Autodesk Inventor part; units mm, degrees
ref_plane "YZ Plane" through (0, 0, 0) normal (1, 0, 0) x (0, 1, 0)
ref_plane "XZ Plane" through (0, 0, 0) normal (0, 1, 0) x (-1, 0, 0)
ref_plane "XY Plane" through (0, 0, 0) normal (0, 0, 1) x (1, 0, 0)
sketch "Sketch1" plane through (0, 0, 0) normal (0, 1, 0) x (-1, 0, 0)
  line L0 (0, 0) -> (-152.4, 0)
  line L1 (-152.4, 0) -> (-152.4, -127)
  line L2 (-152.4, -127) -> (0, -127)
  line L3 (0, -127) -> (0, 0)
  line L4 (0, 0) -> (-152.4, 0)
  line L5 (-152.4, 0) -> (-152.4, 3.175)
  line L6 (-152.4, 3.175) -> (0, 3.175)
  line L7 (0, 3.175) -> (0, 0)
  line L8 (0, -127) -> (-152.4, -127)
  line L9 (-152.4, -127) -> (-152.4, -130.175)
  line L10 (-152.4, -130.175) -> (0, -130.175)
  line L11 (0, -130.175) -> (0, -127)
  dimension "d0" = 152.4
  dimension "d1" = 127
  dimension "d2" = 152.4
  dimension "d3" = 3.175
  dimension "d4" = 152.4
  dimension "d5" = 3.175
extrude "Extrusion1" add sketch "Sketch1" along normal blind 50.8 contours L0 L5 L6 L7 | L11 L10 L9 L2
sketch "Sketch2" plane through (0, 50.8, 0) normal (0, 1, 0) x (1, 0, 0)
  line L0 (0, -3.175) -> (152.4, -3.175)
  line L1 (0, -3.175) -> (-3.175, -3.175)
  line L2 (-3.175, -3.175) -> (-3.175, 130.175)
  line L3 (-3.175, 130.175) -> (0, 130.175)
  line L4 (0, 130.175) -> (0, -3.175)
  point P0 (0, 0)
  dimension "d8" = 3.175
  dimension "d9" = 133.35
extrude "Extrusion2" add sketch "Sketch2" against normal blind 45.72
sketch "Sketch3" plane through (0, 0, 3.175) normal (0, 0, 1) x (1, 0, 0)
  line L0 (-3.175, 5.08) -> (0, 5.08)
  line L1 (-3.175, 5.08) -> (0, 5.08)
  line L2 (0, 5.08) -> (0, 0)
  line L3 (0, 0) -> (-3.175, 0)
  line L4 (-3.175, 0) -> (-3.175, 5.08)
extrude "Extrusion3" add sketch "Sketch3" against normal blind 3.175
sketch "Sketch4" plane through (152.4, 0, -130.175) normal (0, 0, -1) x (-1, 0, 0)
  line L0 (152.4, 0) -> (155.575, 0)
  line L1 (155.575, 0) -> (155.575, 5.08)
  line L2 (155.575, 5.08) -> (152.4, 5.08)
  line L3 (152.4, 5.08) -> (152.4, 0)
extrude "Extrusion4" add sketch "Sketch4" against normal blind 3.175
sketch "Sketch5" plane through (0, 50.8, 0) normal (0, 1, 0) x (1, 0, 0)
  line L0 (152.4, -3.175) -> (152.4, 0)
  line L1 (0, 127) -> (152.4, 127)
  line L2 (152.4, 0) -> (149.225, 0)
  line L3 (149.225, 0) -> (149.225, 127)
  line L4 (149.225, 127) -> (152.4, 127)
  line L5 (152.4, 127) -> (152.4, 0)
  point P0 (0, 0)
  dimension "d16" = 3.175
extrude "Extrusion5" add sketch "Sketch5" against normal blind 45.72
sketch "Sketch7" plane through (0, 0, 0) normal (0, -1, 0) x (1, 0, 0)
  line L0 (-3.175, 3.175) -> (-3.175, 0)
  line L1 (152.4, -127) -> (152.4, 0)
  line L2 (-3.175, 3.175) -> (152.4, 3.175)
  line L3 (152.4, 3.175) -> (152.4, -9.525)
  line L4 (152.4, -9.525) -> (-3.175, -9.525)
  line L5 (-3.175, -9.525) -> (-3.175, 3.175)
  line L6 (-3.175, -130.175) -> (-3.175, 3.175)
  line L7 (-3.175, -130.175) -> (152.4, -130.175)
  line L8 (152.4, -130.175) -> (152.4, -117.475)
  line L9 (152.4, -117.475) -> (-3.175, -117.475)
  line L10 (-3.175, -117.475) -> (-3.175, -130.175)
  point P0 (0, 0)
  point P1 (-3.175, -117.475)
  dimension "d19" = 12.7
  dimension "d20" = 155.575
  dimension "d21" = 12.7
extrude "Extrusion6" add sketch "Sketch7" along normal blind 3.175 contours L2 L3 L1 L4 L5 L0 | L9 L1 L8 L7 L6
sketch "Sketch8" plane through (0, 50.8, 0) normal (0, 1, 0) x (1, 0, 0)
  line L0 (0, 0) -> (49.53, 0) construction
  line L1 (49.53, 0) -> (49.53, 127) construction
  line L2 (49.53, 127) -> (0, 127) construction
  line L3 (0, 127) -> (0, 0) construction
  line L4 (149.225, 0) -> (152.4, 0) construction
  line L5 (149.225, 0) -> (99.695, 0) construction
  line L6 (99.695, 0) -> (99.695, 127) construction
  line L7 (99.695, 127) -> (149.225, 127) construction
  line L8 (149.225, 127) -> (149.225, 0) construction
  line L9 (99.695, 0) -> (96.52, 0)
  line L10 (96.52, 0) -> (96.52, 127)
  line L11 (96.52, 127) -> (99.695, 127)
  line L12 (99.695, 127) -> (99.695, 0)
  line L13 (49.53, 0) -> (52.705, 0)
  line L14 (52.705, 0) -> (52.705, 127)
  line L15 (52.705, 127) -> (49.53, 127)
  line L16 (49.53, 127) -> (49.53, 0)
  dimension "d24" = 49.53
  dimension "d25" = 127
  dimension "d26" = 49.53
  dimension "d27" = 127
  dimension "d28" = 3.175
  dimension "d29" = 127
  dimension "d30" = 3.175
  dimension "d31" = 127
extrude "Extrusion7" add sketch "Sketch8" against normal blind 45.72
sketch "Sketch9" plane through (152.4, 50.8, 3.175) normal (1, 0, 0) x (0, 0, -1)
  line L0 (0, 0) -> (133.35, 0)
  line L1 (133.35, 0) -> (133.35, 50.8)
  line L2 (133.35, 50.8) -> (0, 50.8)
  line L3 (0, 50.8) -> (0, 0)
  line L4 (133.35, 50.8) -> (184.15, 50.8)
  line L5 (184.15, 50.8) -> (133.35, 0)
  line L6 (0, 50.8) -> (-50.8, 50.8)
  line L7 (0, 50.8) -> (50.8, 50.8) construction
  line L8 (-50.8, 50.8) -> (0, 0)
  point P0 (3.175, -50.8)
  dimension "d34" = 133.35
  dimension "d35" = 50.8
  dimension "d36" = 50.8
  dimension "d37" = 50.8
  dimension "d38" = 180
extrude "Extrusion8" add sketch "Sketch9" against normal blind 3.175
sketch "Sketch10" plane through (-3.175, 50.8, -130.175) normal (-1, 0, 0) x (0, 0, 1)
  line L0 (3.175, 0) -> (0, 0)
  line L1 (0, 0) -> (133.35, 0)
  line L2 (133.35, 0) -> (133.35, 50.8)
  line L3 (133.35, 50.8) -> (0, 50.8)
  line L4 (0, 50.8) -> (0, 0)
  line L5 (-50.8, 50.8) -> (184.15, 50.8)
  line L6 (0, 50.8) -> (-50.8, 50.8)
  line L7 (-50.8, 50.8) -> (0, 0)
  line L8 (133.35, 50.8) -> (184.15, 50.8)
  line L9 (133.35, 0) -> (184.15, 50.8)
  point P0 (130.175, -50.8)
  dimension "d41" = 133.35
  dimension "d42" = 50.8
extrude "Extrusion9" add sketch "Sketch10" against normal blind 3.175
sketch "Sketch11" plane through (-3.175, 50.8, 3.175) normal (0, -0.7071, 0.7071) x (1, 0, 0)
  line L0 (0, 71.842) -> (0, -94.2927)
  line L1 (155.575, 0) -> (155.575, -38.1661)
  line L2 (0, 71.842) -> (155.575, 71.842)
  line L3 (155.575, 71.842) -> (155.575, 0)
  line L4 (155.575, 0) -> (0, 0)
  line L5 (0, 0) -> (0, 71.842)
  point P0 (3.175, -38.1661)
  point P1 (0, 0)
extrude "Extrusion10" add sketch "Sketch11" along normal blind 3.175
sketch "Sketch12" plane through (152.4, 50.8, -130.175) normal (0, -0.7071, -0.7071) x (-1, 0, 0)
  line L0 (0, 0) -> (0, 71.842)
  line L1 (152.4, 0) -> (155.575, 0)
  line L2 (0, 71.842) -> (155.575, 71.842)
  line L3 (155.575, 71.842) -> (155.575, 0)
  line L4 (155.575, 0) -> (0, 0)
  line L5 (0, 0) -> (0, 71.842)
  point P0 (152.4, -127.9686)
extrude "Extrusion11" add sketch "Sketch12" along normal blind 3.175
sketch "Sketch13" plane through (-3.175, 101.6, 53.975) normal (0, 1, 0) x (1, 0, 0)
  line L0 (52.705, 180.975) -> (52.705, 53.975) construction
  line L1 (52.705, 53.975) -> (52.705, 0) construction
  line L2 (152.4, 0) -> (3.175, 0) construction
  line L3 (55.88, 53.975) -> (55.88, 180.975) construction
  line L4 (55.88, 180.975) -> (55.88, 234.95) construction
  line L5 (3.175, 234.95) -> (152.4, 234.95) construction
  line L6 (52.705, 0) -> (55.88, 0)
  line L7 (55.88, 0) -> (55.88, 234.95)
  line L8 (55.88, 234.95) -> (52.705, 234.95)
  line L9 (52.705, 234.95) -> (52.705, 0)
  point P0 (3.175, 53.975)
extrude "Extrusion12" add sketch "Sketch13" against normal blind 3.175
sketch "Sketch14" plane through (52.705, 101.6, 53.975) normal (1, 0, 0) x (0, 0, -1)
  line L0 (3.175, -3.175) -> (50.8, -50.8)
  line L1 (50.8, -50.8) -> (50.8, -3.175)
  line L2 (231.775, -3.175) -> (3.175, -3.175)
  point P0 (53.975, -101.6)
extrude "Extrusion13" add sketch "Sketch14" against normal blind 3.175
sketch "Sketch15" plane through (52.705, 101.6, 53.975) normal (1, 0, 0) x (0, 0, -1)
  line L0 (50.8, -50.8) -> (50.8, -3.175)
  line L1 (50.8, -3.175) -> (184.15, -3.175)
  line L2 (184.15, -3.175) -> (184.15, -50.8)
  line L3 (184.15, -50.8) -> (50.8, -50.8)
  line L4 (50.8, -50.8) -> (50.8, -3.175)
  line L5 (184.15, -50.8) -> (231.775, -3.175)
  line L6 (231.775, -3.175) -> (184.15, -3.175)
  line L7 (231.775, -3.175) -> (50.8, -3.175)
  point P0 (53.975, -101.6)
extrude "Extrusion14" add sketch "Sketch15" against normal blind 3.175
sketch "Sketch16" plane through (-3.175, 101.6, 53.975) normal (0, 1, 0) x (1, 0, 0)
  line L0 (152.4, 53.975) -> (102.87, 53.975) construction
  line L1 (102.87, 53.975) -> (102.87, 0) construction
  line L2 (152.4, 0) -> (55.88, 0) construction
  line L3 (55.88, 180.975) -> (99.695, 180.975) construction
  line L4 (99.695, 180.975) -> (99.695, 234.95) construction
  line L5 (55.88, 234.95) -> (152.4, 234.95) construction
  line L6 (102.87, 0) -> (99.695, 0)
  line L7 (99.695, 0) -> (99.695, 234.95)
  line L8 (99.695, 234.95) -> (102.87, 234.95)
  line L9 (102.87, 234.95) -> (102.87, 0)
  point P0 (3.175, 53.975)
extrude "Extrusion15" add sketch "Sketch16" against normal blind 3.175
sketch "Sketch17" plane through (99.695, 101.6, 53.975) normal (1, 0, 0) x (0, 0, -1)
  line L0 (231.775, -3.175) -> (3.175, -3.175)
  line L1 (3.175, -3.175) -> (50.8, -50.8)
  line L2 (50.8, -50.8) -> (50.8, -3.175)
  line L3 (50.8, -3.175) -> (3.175, -3.175)
  line L4 (50.8, -3.175) -> (184.15, -3.175)
  line L5 (184.15, -3.175) -> (184.15, -50.8)
  line L6 (184.15, -50.8) -> (50.8, -50.8)
  line L7 (50.8, -50.8) -> (50.8, -3.175)
  line L8 (184.15, -3.175) -> (231.775, -3.175)
  line L9 (184.15, -50.8) -> (231.775, -3.175)
  point P0 (53.975, -101.6)
extrude "Extrusion16" add sketch "Sketch17" against normal blind 3.175
properties part number "BeadCompartments_2"
Source: CAD feature listing. Evaluate the final solid. Frame: model axes, mm. A direction names the side the tool comes from. Coordinates: 2 decimals unless noted, no trailing zeros. Order: outer loops, then holes, each group sorted by start corner. A loop starts at its lowest first (then second) coordinate and runs counter-clockwise, first axis right, second up. Notation, with made-up numbers: (11, 22) - (56, 22) arc R29 ccw to (56, 43) - close; hole circle Ø2 at (42.5, 46). An arc over 180 degrees is marked (long way). One line per item, written item: value.
1) Cut plane C-C on y = 20. Output: boundary loops of the cut face in (x, z) (3 decimals), plus the area to 3 significant figures.
Computed values:
outline: (-3.175, -130.175) - (152.4, -130.175) - (152.4, 3.175) - (-3.175, 3.175) - close; hole (0, -127) - (49.53, -127) - (49.53, 0) - (0, 0) - close; hole (52.705, -127) - (96.52, -127) - (96.52, 0) - (52.705, 0) - close; hole (99.695, -127) - (149.225, -127) - (149.225, 0) - (99.695, 0) - close
area: 2,600 mm^2
2) Cut plane A-A on z = -58.5. Output: boundary loops of the cut face in (x, y) (3 decimals).
Computed values:
outline: (-3.175, 5.08) - (0, 5.08) - (0, 101.6) - (-3.175, 101.6) - close; (49.53, 5.08) - (52.705, 5.08) - (52.705, 101.6) - (49.53, 101.6) - close; (96.52, 5.08) - (99.695, 5.08) - (99.695, 101.6) - (96.52, 101.6) - close; (149.225, 5.08) - (152.4, 5.08) - (152.4, 101.6) - (149.225, 101.6) - close
3) Contact query for flat-ended pins moving along their axis: pin 1 (3.5 mm diameter, centred on x = 98.5, z = -73, fed in from -Y); pin 2 (1.6 mm diameter, centred on x = 38.5, y = -1, fed in from -Z) (3 decimals); pin 3 (8 mm diameter, centred on x = 45.5, z = -30, fed in from +Y); pin 4 (3.5 mm diameter, centred on x = 82, z = -128.5, fed in from +Y) (3 decimals). Output: stop coordinate, or through.
Computed values:
pin 1: stops at y = 5.08
pin 2: stops at z = -130.175
pin 3: passes through
pin 4: stops at y = 50.875
4) Ray query, line 1 (X direction, y = 72, z = 16) (3 decimals); line 2 (Z direction, x = 145, y = 43.5) (3 decimals); line 3 (Z direction, x = 88.5, y = 57.5) (3 decimals). Return the intervals inside material, ascending. Write a range as [from, to].
Computed values:
line 1: x = [-3.175, 0], [49.53, 52.705], [96.52, 99.695], [149.225, 152.4]
line 2: z = [-130.175, -127], [0, 3.175]
line 3: z = [-141.365, -136.875], [9.875, 14.365]
5) Reachability of faces 1 (the face through (73.523, 74.311, 31.176)), 2 (the face through (74.919, 76.556, -155.931)) from +Z, -Z, +X, -X, +Y, -Y: full face, straight path, thin tool, end or side. Return the list, or none.
Computed values:
face 1: +Z, +X, -X, -Y
face 2: +Y
6) Cut plane D-D on y = 91.5. Output: boundary loops of the cut face in (x, z) (3 decimals).
Computed values:
outline: (-3.175, -175.365) - (152.4, -175.365) - (152.4, 48.365) - (-3.175, 48.365) - close; hole (0, -170.875) - (49.53, -170.875) - (49.53, 43.875) - (0, 43.875) - close; hole (52.705, -170.875) - (96.52, -170.875) - (96.52, 43.875) - (52.705, 43.875) - close; hole (99.695, -170.875) - (149.225, -170.875) - (149.225, 43.875) - (99.695, 43.875) - close
7) Mould query, pull axis X, two halves, no side actions, for faces 3 (the face through (-3.175, 45, -63)), 4 (the face through (99.695, 65, -65)), 5 (the face through (49.53, 65, -62)), 6 (the face through (74, 0, -5)). Classes: released by +X, released by -X, zero draft, split by the parting line, or undercut.
Computed values:
face 3: released by -X
face 4: undercut
face 5: undercut
face 6: zero draft
